Source: three-view drawing plus pictorial views. Frame: mm from the lowest corner of the part. A direction names the side the tool comes from. Give positions to 0.01 mm unless a question says otherwise; leave off trailing zeros. Order: outer loops, then holes, each group sorted by start corner. A loop starts at its lowest first (then second) coordinate and runs counter-clockwise, first axis right, second up. Notation, with made-up numbers: (-19, -2) -> (13, -2) arc R5 ccw to (13, 4) -> close; hole circle Ø2 at (24.5, 82). An arc over 180 degrees is marked (long way). Answer in a Markdown table with one row per item.
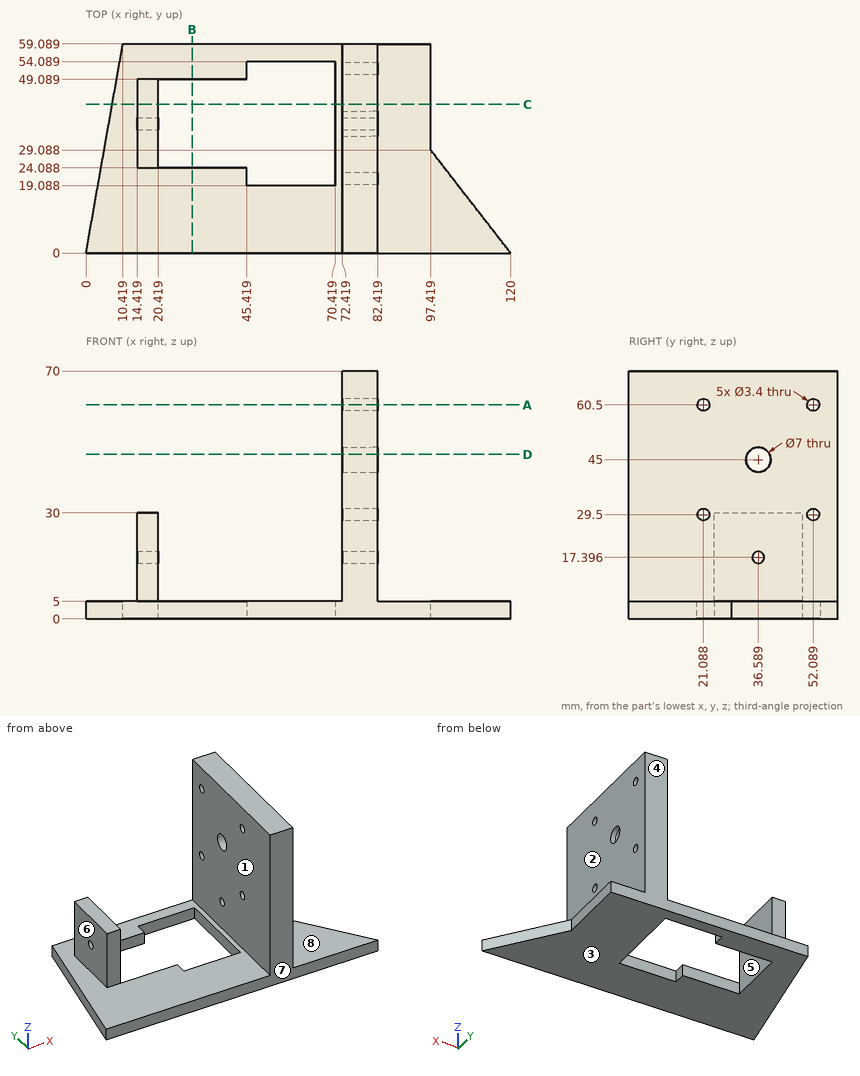
(1) Access query for the marked faces 4, 5, 6, 7 and 8. Directions: +Z, -Z, +X, -X, +Y, -Y. A direction counts if a zero-diameter tool reaches every point of the face in a straight line with its end or side. Return the directions, or none.
A:
| item | result |
|---|---|
| face 4 | +Z, -Z, +X, -X, +Y |
| face 5 | +Z, -Z |
| face 6 | +Z, -X, +Y, -Y |
| face 7 | +Z, -Z, +X, -X, -Y |
| face 8 | +Z, +X, +Y, -Y |
(2) Ray query, probe 1 along Y at (x, z) = (76.5, 60.5); probe 2 along X at (y, z) = (27, 17); probe 3 along Z at (x, y) = (74, 37) (1 decimal). Return the intervals inside material, ascending.
A:
| item | result |
|---|---|
| probe 1 | y = 0 to 19.39, 22.79 to 50.39, 53.79 to 59.09 |
| probe 2 | x = 14.42 to 20.42, 72.42 to 82.42 |
| probe 3 | z = 0 to 15.7, 19 to 41.5, 48.5 to 70 |
(3) Section query D-D (z = 46.5). Return the cut outline in (x, y).
A:
| item | result |
|---|---|
| outline | (72.42, 0) -> (82.42, 0) -> (82.42, 33.43) -> (72.42, 33.43) -> close; (72.42, 39.75) -> (82.42, 39.75) -> (82.42, 59.09) -> (72.42, 59.09) -> close |
(4) Pull-direction query (X, two-part tool) for the marked faces 1, 2 and 3; classes: +X half, -X half, draft (parallel to the pull), parting line (faces both ways), or undercut.
A:
| item | result |
|---|---|
| face 1 | undercut |
| face 2 | +X half |
| face 3 | draft |
(5) Section query C-C (y = 42). Return the cut outline in (x, z) (1 decimal), plus the area to 3 significant figures.
A:
| item | result |
|---|---|
| outline | (7.4, 0) -> (20.4, 0) -> (20.4, 30) -> (14.4, 30) -> (14.4, 5) -> (7.4, 5) -> close; (70.4, 0) -> (97.4, 0) -> (97.4, 5) -> (82.4, 5) -> (82.4, 70) -> (72.4, 70) -> (72.4, 5) -> (70.4, 5) -> close |
| area | 1,000 mm^2 |
(6) Section query A-A (z = 60.5). Return the cut outline in (x, y).
A:
| item | result |
|---|---|
| outline | (72.42, 0) -> (82.42, 0) -> (82.42, 19.39) -> (72.42, 19.39) -> close; (72.42, 22.79) -> (82.42, 22.79) -> (82.42, 50.39) -> (72.42, 50.39) -> close; (72.42, 53.79) -> (82.42, 53.79) -> (82.42, 59.09) -> (72.42, 59.09) -> close |
(7) Section query B-B (x = 30). Return the cut outline in (y, z).
A:
| item | result |
|---|---|
| outline | (0, 0) -> (24.09, 0) -> (24.09, 5) -> (0, 5) -> close; (49.09, 0) -> (59.09, 0) -> (59.09, 5) -> (49.09, 5) -> close |
(8) First-contact query: pin 1 Ø5.5 at (y, z) = (40, 3.5) entering from +X; pin 2 Ø11 at (y, z) = (36.59, 45) entering from -X; pin 3 Ø1.8 at (x, z) = (18.5, 13.5) entering from -Y. Flat tips, straight axial feed; report the tip coordinate or a pass-through.
A:
| item | result |
|---|---|
| pin 1 | stops at x = 97.42 |
| pin 2 | stops at x = 72.42 |
| pin 3 | stops at y = 24.09 |
